Build history of the part. All positions in model axes, mm. Give positions to 0.01 mm unless a question says otherwise; leave off trailing zeros. Order: outer loops, then holes, each group sorted by start corner. A loop starts at its lowest first (then second) coordinate and runs counter-clockwise, first axis right, second up. Notation, with made-up numbers: (41.25, -31) - (62.25, -31) arc R29 cw to (62.25, -9) - close; hole circle Ø4 at (47, 68.25). An arc over 180 degrees is marked (long way). Write each question's results on one line, items separated by ' | '. Start each with the question number.
1) Cut at B-B on x = -7. List the corners of the cut face in (y, z).
2) Two-plate mould, pull along Y, no slides. Class faces 1 (the face through (-1, 18, 0)), 2 (the face through (43, 15, 1)): +Y half, -Y half, draft (parallel to the pull), parting line (faces both ways), or undercut.
3) Drop flat-ended pins along their axis: pin 1 Ø0.6 at (y, z) = (-38.5, 1.5) entering from +X; pin 2 Ø0.6 at (y, z) = (39.5, 0.5) entering from -X; pin 3 Ø1 at (x, z) = (-74, 1) entering from -Y. Give the stop position or say it passes through.
4) Cut at D-D on y = 0. List the corners of the cut face in (x, z), plus the area to 3 significant figures.
5) Drill centre lines: line 1 along Y through (x, z) = (47, 1); line 2 along X through (y, z) = (4.5, 1.75); line 3 along Y through (x, z) = (19, 0.9). Where is each one in solid material? Low to high. Write a range as from..to.
6) Cut at A-A on y = 9. List the corners of the cut face in (x, z), plus the area to 3 significant figures.
7) Cut at C-C on x = 47. List the corners of the cut face in (y, z), plus the area to 3 significant figures.
Solid Edge part; units mm, degrees
sketch "Sketch1" plane through (0, 0, 0) normal (0, 0, 1) x (1, 0, 0)
  line L0 (77, -40) -> (77, 40)
  line L1 (77, 40) -> (-77, 40)
  line L2 (-77, 40) -> (-77, -40)
  line L3 (-77, -40) -> (77, -40)
extrude "Protrusion1" add sketch "Sketch1" along normal blind 2
sketch "Sketch2" plane through (0, 0, 0) normal (0, 0, 1) x (1, 0, 0)
  line L0 (-77, 38) -> (-65, 38)
  line L1 (-65, 38) -> (-65, 40)
  line L2 (-65, 40) -> (-77, 40)
  line L3 (-77, 40) -> (-77, 38)
  line L4 (-55, 38) -> (-35, 38)
  line L5 (-35, 38) -> (-35, 40)
  line L6 (-35, 40) -> (-55, 40)
  line L7 (-55, 40) -> (-55, 38)
  line L8 (-25, 38) -> (-5, 38)
  line L9 (-5, 38) -> (-5, 40)
  line L10 (-5, 40) -> (-25, 40)
  line L11 (-25, 40) -> (-25, 38)
  line L12 (5, 38) -> (25, 38)
  line L13 (25, 38) -> (25, 40)
  line L14 (25, 40) -> (5, 40)
  line L15 (5, 40) -> (5, 38)
  line L16 (35, 38) -> (55, 38)
  line L17 (55, 38) -> (55, 40)
  line L18 (55, 40) -> (35, 40)
  line L19 (35, 40) -> (35, 38)
  line L20 (65, 38) -> (77, 38)
  line L21 (77, 40) -> (77, 38)
  line L22 (77, 40) -> (65, 40)
  line L23 (65, 40) -> (65, 38)
  line L24 (73, 25) -> (73, 15)
  line L25 (73, 15) -> (75, 15)
  line L26 (75, 15) -> (75, 25)
  line L27 (75, 25) -> (73, 25)
  line L28 (73, 5) -> (73, -5)
  line L29 (73, -5) -> (75, -5)
  line L30 (75, -5) -> (75, 5)
  line L31 (75, 5) -> (73, 5)
  line L32 (73, -15) -> (73, -25)
  line L33 (73, -25) -> (75, -25)
  line L34 (75, -25) -> (75, -15)
  line L35 (75, -15) -> (73, -15)
  line L36 (77, -38) -> (65, -38)
  line L37 (65, -38) -> (65, -40)
  line L38 (65, -40) -> (77, -40)
  line L39 (77, -38) -> (77, -40)
  line L40 (55, -38) -> (35, -38)
  line L41 (35, -38) -> (35, -40)
  line L42 (35, -40) -> (55, -40)
  line L43 (55, -40) -> (55, -38)
  line L44 (25, -38) -> (5, -38)
  line L45 (5, -38) -> (5, -40)
  line L46 (5, -40) -> (25, -40)
  line L47 (25, -40) -> (25, -38)
  line L48 (-5, -38) -> (-25, -38)
  line L49 (-25, -38) -> (-25, -40)
  line L50 (-25, -40) -> (-5, -40)
  line L51 (-5, -40) -> (-5, -38)
  line L52 (-35, -38) -> (-55, -38)
  line L53 (-55, -38) -> (-55, -40)
  line L54 (-55, -40) -> (-35, -40)
  line L55 (-35, -40) -> (-35, -38)
  line L56 (-65, -38) -> (-77, -38)
  line L57 (-77, -40) -> (-77, -38)
  line L58 (-77, -40) -> (-65, -40)
  line L59 (-65, -40) -> (-65, -38)
  line L60 (-73, -25) -> (-73, -15)
  line L61 (-73, -15) -> (-75, -15)
  line L62 (-75, -15) -> (-75, -25)
  line L63 (-75, -25) -> (-73, -25)
  line L64 (-73, -5) -> (-73, 5)
  line L65 (-73, 5) -> (-75, 5)
  line L66 (-75, 5) -> (-75, -5)
  line L67 (-75, -5) -> (-73, -5)
  line L68 (-73, 15) -> (-73, 25)
  line L69 (-73, 25) -> (-75, 25)
  line L70 (-75, 25) -> (-75, 15)
  line L71 (-75, 15) -> (-73, 15)
extrude "ExtrudedCutout_1" cut sketch "Sketch2" along normal blind 2
sketch "Sketch3" plane through (0, 0, 0) normal (0, 0, 1) x (1, 0, 0)
  line L0 (19.95, 17) -> (-19.95, 17)
  line L1 (-19.95, 17) -> (-19.95, -17)
  line L2 (-19.95, -17) -> (19.95, -17)
  line L3 (19.95, -17) -> (19.95, 17)
extrude "ExtrudedCutout_2" cut sketch "Sketch3" along normal blind 2
sketch "Sketch4" plane through (0, 0, 0) normal (0, 0, 1) x (1, 0, 0)
  line L0 (-11.35, 22.5) -> (-21.35, 22.5)
  line L1 (-21.35, 22.5) -> (-21.35, 19.5)
  line L2 (-21.35, 19.5) -> (-11.35, 19.5)
  line L3 (-11.35, 19.5) -> (-11.35, 22.5)
  line L4 (21.65, 22.5) -> (11.65, 22.5)
  line L5 (11.65, 22.5) -> (11.65, 19.5)
  line L6 (11.65, 19.5) -> (21.65, 19.5)
  line L7 (21.65, 19.5) -> (21.65, 22.5)
  line L8 (-11.35, -19) -> (-21.35, -19)
  line L9 (-21.35, -19) -> (-21.35, -22)
  line L10 (-21.35, -22) -> (-11.35, -22)
  line L11 (-11.35, -22) -> (-11.35, -19)
  line L12 (21.65, -19) -> (11.65, -19)
  line L13 (11.65, -19) -> (11.65, -22)
  line L14 (11.65, -22) -> (21.65, -22)
  line L15 (21.65, -22) -> (21.65, -19)
extrude "ExtrudedCutout_3" cut sketch "Sketch4" along normal blind 2
sketch "Sketch5" plane through (0, 0, 0) normal (0, 0, 1) x (1, 0, 0)
  circle A0 centre (47, 15) radius 4
  circle A1 centre (47, 0) radius 4
  circle A2 centre (47, -15) radius 4
  circle A3 centre (-53, 0) radius 3.5
extrude "ExtrudedCutout_7" cut sketch "Sketch5" along normal blind 2
fillet "Round_1" radius 1 4 edges at (-77, -38, 1) (-77, 38, 1) (77, -38, 1) (77, 38, 1)
properties material "Acrylic, high impact grade"
Results:
1) outline: (-38, 0) - (-17, 0) - (-17, 2) - (-38, 2) - close; (17, 0) - (38, 0) - (38, 2) - (17, 2) - close
2) face 1: draft | face 2: undercut
3) pin 1: x = 65 | pin 2: x = -65 | pin 3: y = -38
4) outline: (-77, 0) - (-75, 0) - (-75, 2) - (-77, 2) - close; (-73, 0) - (-56.5, 0) - (-56.5, 2) - (-73, 2) - close; (-49.5, 0) - (-19.95, 0) - (-19.95, 2) - (-49.5, 2) - close; (19.95, 0) - (43, 0) - (43, 2) - (19.95, 2) - close; (51, 0) - (73, 0) - (73, 2) - (51, 2) - close; (75, 0) - (77, 0) - (77, 2) - (75, 2) - close | area: 190 mm^2
5) line 1: -38..-19, -11..-4, 4..11, 19..38 | line 2: -77..-75, -73..-19.95, 19.95..73, 75..77 | line 3: -38..-22, -19..-17, 17..19.5, 22.5..38
6) outline: (-77, 0) - (-19.95, 0) - (-19.95, 2) - (-77, 2) - close; (19.95, 0) - (77, 0) - (77, 2) - (19.95, 2) - close | area: 228 mm^2
7) outline: (-38, 0) - (-19, 0) - (-19, 2) - (-38, 2) - close; (-11, 0) - (-4, 0) - (-4, 2) - (-11, 2) - close; (4, 0) - (11, 0) - (11, 2) - (4, 2) - close; (19, 0) - (38, 0) - (38, 2) - (19, 2) - close | area: 104 mm^2
